Part model, mm, in its own coordinate system. A direction names the side the tool comes from. Coordinates: 2 decimals unless noted, no trailing zeros. Write each loop counter-clockwise with the first axis right and the second up, starting at its lowest first coordinate (ties: lowest second). Pieces come first, ordered by that corner, then holes. Notation, with made-up numbers: (84, 37) -> (132, 37) arc R22 ccw to (132, 47) -> close; hole circle Ø7 at (19.25, -19). An arc over 180 degrees is marked (long way). Write item = value, one per line.
from build123d import *

# Parameters (mm, degrees)
F0_W          = 41.91
F0_H          = 41.91
F1_DEPTH      = 2.54
F2_W          = 44.45
F2_H          = 44.45
F3_DEPTH      = 2.54
F3_DEPTH_BACK = 19.05
F5_W          = 7.62
F5_H          = 1.27
F6_DEPTH      = 19.05


with BuildPart() as f1:
    # F0 (on Top) → F1 (new body)
    with BuildSketch(Plane.XY):
        with Locations((20.955, 20.955)):
            Rectangle(F0_W, F0_H)
    extrude(amount=F1_DEPTH)

    # F2 (on face) → F3 (join, two sides)
    with BuildSketch(Plane.XY.offset(2.54)) as f3_sk:
        with Locations((20.955, 20.955)):
            Rectangle(F2_W, F2_H)
        Polygon((0, 0), (0, 41.91), (20.955, 41.91), (41.91, 41.91), (41.91, 0), align=None, mode=Mode.SUBTRACT)
    extrude(amount=-F3_DEPTH)
    extrude(f3_sk.sketch, amount=F3_DEPTH_BACK)


with BuildPart() as f4_1:
    # F4: copy of F1
    add(f1.part)


with BuildPart() as f6_tool:
    # F5 (on face) → F6 (new body)
    with BuildSketch(Plane.XY.offset(21.59)):
        with Locations((20.955, 42.545)):
            Rectangle(F5_W, F5_H)
    extrude(amount=-F6_DEPTH)


with BuildPart() as f1_1:
    add(f1.part)

    # F6: cut by f6_tool
    add(f6_tool.part, mode=Mode.SUBTRACT)


with BuildPart() as f4_1_1:
    add(f4_1.part)

    # F6: cut by f6_tool
    add(f6_tool.part, mode=Mode.SUBTRACT)


solid = f1_1.part
Q1. Pin check, flat tip, straight feed: pin 1 (5 mm diameter, centred on x = 7, y = 22.5, fed in from +Z). Stop position of the tip, or through.
Model answer:
pin_1 = 2.54
Q2. Saw through at D-D on x = 22.5. Give the cut face in (y, z), and give its area (3 significant figures).
Model answer:
outline = (-1.27, 0) -> (43.18, 0) -> (43.18, 2.54) -> (0, 2.54) -> (0, 21.59) -> (-1.27, 21.59) -> close
area = 137 mm²
Q3. Probe line 1 (Y direction, x = 16.5, z = 11.25); line 2 (Z direction, x = 13, y = 7.5). List the from-to ranges inside material, lowest first. Write a range as from..to.
Model answer:
line_1 = -1.27..0, 41.91..43.18
line_2 = 0..2.54
Q4. Mould opens along Y. For faces 1 (the face through (20.9, -0.3, 21.59)), 2 (the face through (0, 21, 12)), 3 (the face through (26, 43.18, 11)) say: released by +Y, released by -Y, zero draft, split by the parting line, or undercut.
Model answer:
face_1 = zero draft
face_2 = undercut
face_3 = released by +Y
Q5. Saw through at A-A on x = 34. Give the cut face in (y, z).
Model answer:
outline = (-1.27, 0) -> (43.18, 0) -> (43.18, 21.59) -> (41.91, 21.59) -> (41.91, 2.54) -> (0, 2.54) -> (0, 21.59) -> (-1.27, 21.59) -> close
Q6. Which spindle directions (+Z, -Z, +X, -X, +Y, -Y) get a long thin tool onto all of the face, cutting with end or side? Do faces 4 (the face through (17.145, 43, 12)), 5 (the face through (21, 21, 0)), 6 (the face through (21, 0, 12)). Say none if no direction does.
Model answer:
face_4 = +Z, +Y
face_5 = -Z, +X, -X, +Y, -Y
face_6 = +Z
Q7. Saw through at C-C on z = 6.5. Give the cut face in (x, y) (3 decimals).
Model answer:
outline = (-1.27, -1.27) -> (43.18, -1.27) -> (43.18, 43.18) -> (24.765, 43.18) -> (24.765, 41.91) -> (41.91, 41.91) -> (41.91, 0) -> (0, 0) -> (0, 41.91) -> (17.145, 41.91) -> (17.145, 43.18) -> (-1.27, 43.18) -> close
